CAD build for the part. Positions are in the model's coordinates, mm. Give positions to 0.01 mm unless a question says otherwise; leave off trailing zeros. Write each loop counter-clockwise with the first axis right and the second up, starting at its lowest first coordinate (ties: lowest second). Pieces come first, ordered by that corner, then holes. Notation, with made-up numbers: (-19, 0) -> (-14, 0) arc R32 ccw to (-14, 36) -> close; hole circle Ø6 at (63, 85.25). An arc over 180 degrees is marked (long way). Answer as a JSON object with one key per item and string values.
```python
from build123d import *

# Parameters (mm, degrees)
F0_W     = 108.930484
F0_H     = 85.066848
F0_R     = 24.8637
F1_DEPTH = 85.53001


with BuildPart() as f1:
    # F0 (on Right) → F1 (new body)
    with BuildSketch(Plane.YZ):
        Rectangle(F0_W, F0_H)
        Circle(F0_R, mode=Mode.SUBTRACT)
    extrude(amount=-F1_DEPTH)


solid = f1.part
```
1) Wall check: probe 1 along Z at (x, y) = (-24.5, -13.5); probe 2 along Z at (x, y) = (-9, -15.5); probe 3 along Y at (x, z) = (-71, -23). Give the ranges that are in metal, low to high.
Model answer:
{"probe 1": "z = -42.53 to -20.88, 20.88 to 42.53", "probe 2": "z = -42.53 to -19.44, 19.44 to 42.53", "probe 3": "y = -54.47 to -9.44, 9.44 to 54.47"}
2) Slice it at C-C (x = -15). List the corners of the cut face in (y, z), then the cut area to 3 significant figures.
Model answer:
{"outline": "(-54.47, -42.53) -> (54.47, -42.53) -> (54.47, 42.53) -> (-54.47, 42.53) -> close; hole circle Ø49.73 at (0, 0)", "area": "7,320 mm2"}
3) Slice it at B-B (y = 0). List the corners of the cut face in (x, z).
Model answer:
{"outline": "(-85.53, -42.53) -> (0, -42.53) -> (0, -24.86) -> (-85.53, -24.86) -> close; (-85.53, 24.86) -> (0, 24.86) -> (0, 42.53) -> (-85.53, 42.53) -> close"}
4) Mould opens along Y. For faces 1 (the flat face through (-85.53, -25, 1)), 2 (the cylindrical face through (-42.17, -18.33, 16.8)), 3 (the flat face through (-42, 54.465, -1)) say: released by +Y, released by -Y, zero draft, split by the parting line, or undercut.
Model answer:
{"face 1": "zero draft", "face 2": "undercut", "face 3": "released by +Y"}
5) Slice it at A-A (z = 0). List the corners of the cut face in (x, y).
Model answer:
{"outline": "(-85.53, -54.47) -> (0, -54.47) -> (0, -24.86) -> (-85.53, -24.86) -> close; (-85.53, 24.86) -> (0, 24.86) -> (0, 54.47) -> (-85.53, 54.47) -> close"}
